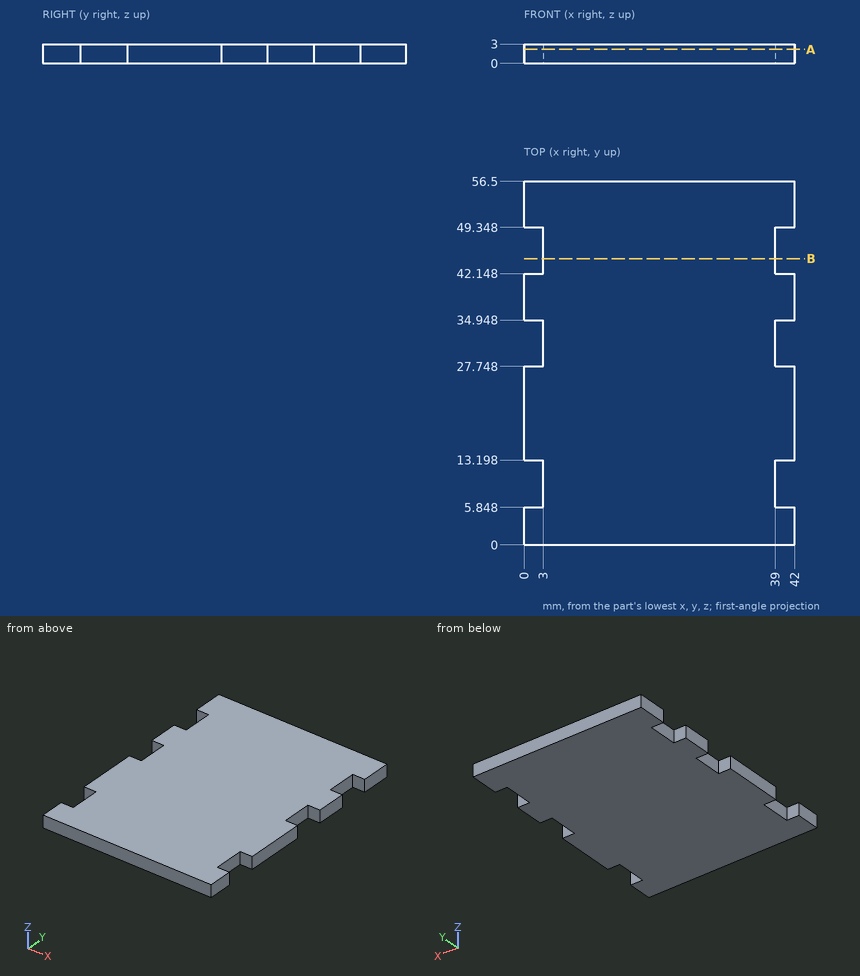
Can you work these out from the drawing? Everything is in mm from the part's minimum corner. Coordinates: 2 decimals unless noted, no trailing zeros. Loops run counter-clockwise (first coordinate to the right, second up) from the corner with the lowest first, then second, coordinate; pieces in that order, holes last.
1) For pin 1 (0.9 mm diameter, centred on y = 32.5, z = 1.5, fed in from +X); pin 2 (0.9 mm diameter, centred on y = 11, z = 1.5, fed in from -X), each with a flat end and sliding along its axis, tell me the tip position at first contact or that it passes through.
2) I need wall thicknesses on probe 1 along X at (y, z) = (9.5, 2.4). Which ranges of the line are inside material? Lowest first, please.
3) Imagine slicing it at B-B on y = 44.5. List the corners of the cut face in (x, z) for me.
4) Imagine slicing it at A-A on z = 2.15. List the corners of the cut face in (x, y) for me, plus the area to 3 significant figures.
Completed:
1. pin 1: stops at x = 39
1. pin 2: stops at x = 3
2. probe 1: x = 3 to 39
3. outline: (3, 0) - (39, 0) - (39, 3) - (3, 3) - close
4. outline: (0, 0) - (42, 0) - (42, 5.85) - (39, 5.85) - (39, 13.2) - (42, 13.2) - (42, 27.75) - (39, 27.75) - (39, 34.95) - (42, 34.95) - (42, 42.15) - (39, 42.15) - (39, 49.35) - (42, 49.35) - (42, 56.5) - (0, 56.5) - (0, 49.35) - (3, 49.35) - (3, 42.15) - (0, 42.15) - (0, 34.95) - (3, 34.95) - (3, 27.75) - (0, 27.75) - (0, 13.2) - (3, 13.2) - (3, 5.85) - (0, 5.85) - close
4. area: 2,240 mm2
